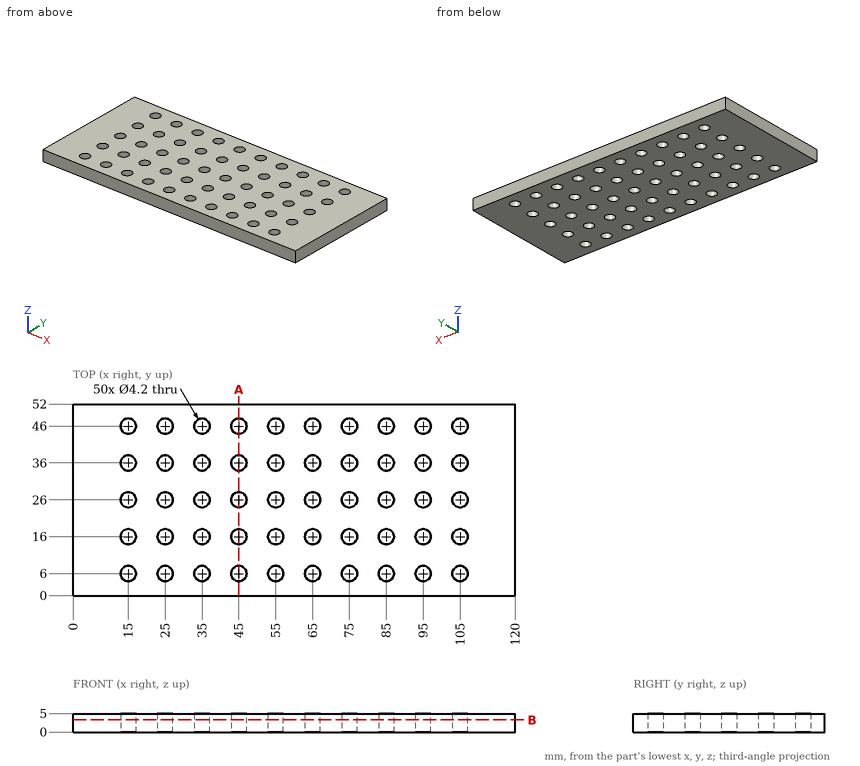
Job drawing, mm, ordinate dimensions from the low corner. One solid piece. Give positions to 0.01 mm unless a question says otherwise; leave off trailing zeros. Loops run counter-clockwise (first coordinate to the right, second up) from the corner with the lowest first, then second, coordinate; pieces in that order, holes last. Notation, with made-up numbers: (60.5, -18.5) - (114.5, -18.5) arc R32 cw to (114.5, 19.5) - close; hole circle Ø8 at (-1, 16). An arc over 180 degrees is marked (long way). Use one line per item in the form item = value.
(1) Cut at A-A (x = 45). Give the cut face in (y, z).
Determined:
outline = (0, 0) - (3.9, 0) - (3.9, 5) - (0, 5) - close; (8.1, 0) - (13.9, 0) - (13.9, 5) - (8.1, 5) - close; (18.1, 0) - (23.9, 0) - (23.9, 5) - (18.1, 5) - close; (28.1, 0) - (33.9, 0) - (33.9, 5) - (28.1, 5) - close; (38.1, 0) - (43.9, 0) - (43.9, 5) - (38.1, 5) - close; (48.1, 0) - (52, 0) - (52, 5) - (48.1, 5) - close
(2) Drill centre lines: L1, parallel to Y at x = 75, z = 2.2; L2, parallel to Y at x = 76.5, z = 2.15. Where is each one in solid material? Low to high.
Determined:
L1 = 0 to 3.9, 8.1 to 13.9, 18.1 to 23.9, 28.1 to 33.9, 38.1 to 43.9, 48.1 to 52
L2 = 0 to 4.53, 7.47 to 14.53, 17.47 to 24.53, 27.47 to 34.53, 37.47 to 44.53, 47.47 to 52
(3) Drop a flat-ended pin along its axis: P1, Ø3.5, axis at x = 85, y = 26, coming from the -Z side. Give the stop position or say it passes through.
Determined:
P1 = through
(4) Cut at B-B (z = 3.35). Count the separate pieces of the cut face and the enclosed holes in it, then the cut area to 3 significant figures.
Determined:
separate_pieces = 1
enclosed_holes = 50
area = 5,550 mm^2
